Source: CAD feature listing. Evaluate the final solid. Frame: model axes, mm. Face numbers are marked on the shaded views. A direction names the side the tool comes from. Give positions to 0.01 mm unless a question says otherwise; leave off trailing zeros. Loops run counter-clockwise (first coordinate to the right, second up) from the corner with the lowest first, then second, coordinate; pieces in that order, holes last. Notation, with made-up numbers: M 29,-21.75 L 82,-21.75 A32 ccw 82,5.25 Z; hole C -34,45 d1. An arc over 180 degrees is marked long. Write item = value, one per line.
from build123d import *

# Parameters (mm, degrees)
ESQUISSE1_W                              = 45
ESQUISSE1_H                              = 35
BOSS_EXTRU_1_DEPTH                       = 2
ESQUISSE2_W                              = 35
ESQUISSE2_H                              = 32
BOSS_EXTRU_2_DEPTH                       = 1
CONG_1_R                                 = 5
CONG_2_R                                 = 0.5
CHANFREIN1_SIZE                          = 0.5
ESQUISSE3_R                              = 1.75
ENL_V_MAT_EXTRU_1_DEPTH                  = 29.574464124
DIAM_TRE_DU_PER_AGE_6_5_6_5_1_D          = 6.5
DIAM_TRE_DU_PER_AGE_6_5_6_5_1_DEPTH      = 1
FRAISAGE_POUR_VIS_T_TE_FRAIS_E_6_2_COUNT = 2
FRAISAGE_POUR_VIS_T_TE_FRAIS_E_6_2_PITCH = 33.301651611
FRAISAGE_POUR_VIS_T_TE_FRAIS_E_6_3_COUNT = 2
FRAISAGE_POUR_VIS_T_TE_FRAIS_E_6_3_PITCH = 22
FRAISAGE_POUR_VIS_T_TE_FRAIS_E_6_4_COUNT = 2
FRAISAGE_POUR_VIS_T_TE_FRAIS_E_6_4_PITCH = 25


with BuildPart() as part:
    # Esquisse1 → Boss.-Extru.1 (new body)
    with BuildSketch(Plane(origin=(0, 0, 0), x_dir=(1, 0, 0), z_dir=(0, 1, 0))):
        Rectangle(ESQUISSE1_W, ESQUISSE1_H)
    extrude(amount=BOSS_EXTRU_1_DEPTH)

    # Esquisse2 → Boss.-Extru.2 (add)
    with BuildSketch(Plane.XZ):
        Rectangle(ESQUISSE2_W, ESQUISSE2_H)
    extrude(amount=BOSS_EXTRU_2_DEPTH)

    # Congé1
    cong_1_edges = [part.edges().sort_by_distance(p)[0] for p in [
        (17.5, -0.5, -16),
        (17.5, -0.5, 16),
        (-17.5, -0.5, 16),
        (-17.5, -0.5, -16),
    ]]
    fillet(cong_1_edges, radius=CONG_1_R)

    # Congé2
    cong_2_edges = [part.edges().sort_by_distance(p)[0] for p in [
        (22.5, 1, 17.5),
        (-22.5, 1, 17.5),
        (-22.5, 1, -17.5),
        (22.5, 1, -17.5),
    ]]
    fillet(cong_2_edges, radius=CONG_2_R)

    # Chanfrein1
    chanfrein1_edges = [part.edges().sort_by_distance(p)[0] for p in [
        (0, -1, 16),
        (17.5, -1, 0),
        (-17.5, -1, 0),
        (0, -1, -16),
        (-16.035533906, -1, 14.535533906),
        (16.035533906, -1, -14.535533906),
        (-16.035533906, -1, -14.535533906),
        (16.035533906, -1, 14.535533906),
    ]]
    chamfer(chanfrein1_edges, length=CHANFREIN1_SIZE)

    # Esquisse3 → Enlèv. mat.-Extru.1 (cut, through all)
    with BuildSketch(Plane.XZ):
        with Locations(Location((-20, 10, 0), (0, 0, 270))):
            Circle(ESQUISSE3_R)
        with Locations(Location((20, 10, 0), (0, 0, 270))):
            Circle(ESQUISSE3_R)
        with Locations(Location((20, -10, 0), (0, 0, 270))):
            Circle(ESQUISSE3_R)
        with Locations(Location((-20, -10, 0), (0, 0, 270))):
            Circle(ESQUISSE3_R)
    extrude(amount=-ENL_V_MAT_EXTRU_1_DEPTH, mode=Mode.SUBTRACT)

    # Diamètre du perçage Ø6.5 (6.5)1
    with Locations(Plane(origin=(0, 2, 0), x_dir=(1, 0, 0), z_dir=(0, 1, 0))):
        with Locations((-12.5, -11), (12.5, 11), (-12.5, 11), (12.5, -11)):
            Hole(DIAM_TRE_DU_PER_AGE_6_5_6_5_1_D / 2, depth=DIAM_TRE_DU_PER_AGE_6_5_6_5_1_DEPTH)

    # Esquisse4 → Fraisage pour vis à tête fraisée à 6 pans creux M31 (revolve, cut)
    with BuildSketch(Plane(origin=(-12.5, 1, -11), x_dir=(0, 0, 1), z_dir=(1, 0, 0))):
        Polygon((0, 0), (0, 2), (1.7, 2), (1.7, 1.55), (3.25, 0), align=None)
    fraisage_pour_vis_t_te_frais_e_6_pan = revolve(axis=Axis((-12.5, 7.35, -11), (0, -1, 0)), mode=Mode.SUBTRACT)

    # Fraisage pour vis _ t_te frais_e _ 6 2: Fraisage pour vis à tête fraisée à 6 pans creux M31 ×2
    with Locations(*[Vector(0.7507135169227553, 0, 0.6606278948920248) * (i * FRAISAGE_POUR_VIS_T_TE_FRAIS_E_6_2_PITCH) for i in range(1, FRAISAGE_POUR_VIS_T_TE_FRAIS_E_6_2_COUNT)]):
        add(fraisage_pour_vis_t_te_frais_e_6_pan, mode=Mode.SUBTRACT)

    # Fraisage pour vis _ t_te frais_e _ 6 3: Fraisage pour vis à tête fraisée à 6 pans creux M31 ×2
    with Locations(*[(0, 0, i * FRAISAGE_POUR_VIS_T_TE_FRAIS_E_6_3_PITCH) for i in range(1, FRAISAGE_POUR_VIS_T_TE_FRAIS_E_6_3_COUNT)]):
        add(fraisage_pour_vis_t_te_frais_e_6_pan, mode=Mode.SUBTRACT)

    # Fraisage pour vis _ t_te frais_e _ 6 4: Fraisage pour vis à tête fraisée à 6 pans creux M31 ×2
    with Locations(*[(i * FRAISAGE_POUR_VIS_T_TE_FRAIS_E_6_4_PITCH, 0, 0) for i in range(1, FRAISAGE_POUR_VIS_T_TE_FRAIS_E_6_4_COUNT)]):
        add(fraisage_pour_vis_t_te_frais_e_6_pan, mode=Mode.SUBTRACT)


solid = part.part
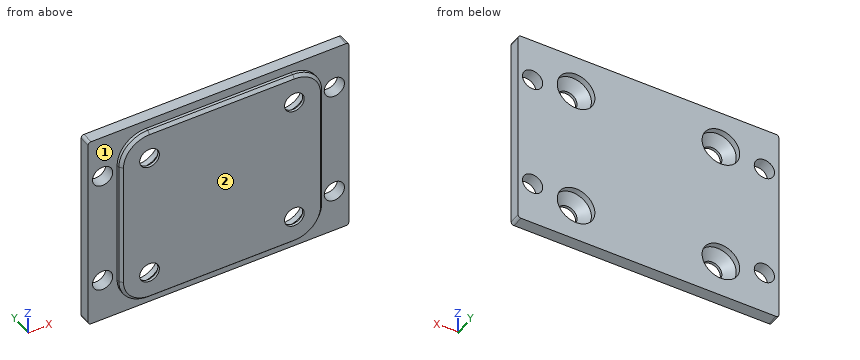
1. Material intervals for probe 1 along Z at (x, y) = (-12.5, -0.75); probe 2 along Z at (x, y) = (-13.5, -0.25); probe 3 along X at (y, z) = (1.6, 10), sorted ascending. Write a range as from..to.
Derived:
probe_1 = -15.75..-12.7, -9.3..9.3, 12.7..15.75
probe_2 = -15.9..-12.73, -9.27..9.27, 12.73..15.9
probe_3 = -22.5..-21.75, -18.25..-15.59, -9.41..9.41, 15.59..18.25, 21.75..22.5
2. Cut plane A-A, the plane x = -20. Return the cut outline in (y, z).
Derived:
outline = M 0,-17.5 L 2,-17.5 L 2,-11.75 L 0,-11.75 Z; M 0,-8.25 L 2,-8.25 L 2,8.25 L 0,8.25 Z; M 0,11.75 L 2,11.75 L 2,17.5 L 0,17.5 Z
3. Cut plane B-B, the plane x = 7. Return the cut outline in (y, z), then the cut area to 3 significant figures.
Derived:
outline = M -1,-15.5 L -0.5,-16 L 0,-16 L 0,-17.5 L 2,-17.5 L 2,17.5 L 0,17.5 L 0,16 L -0.5,16 L -1,15.5 Z
area = 102 mm²
4. First-contact query: pin 1 Ø4 at (x, z) = (20, 10) entering from -Y; pin 2 Ø2 at (x, z) = (-20, -10) entering from +Y; pin 3 Ø10.5 at (x, z) = (12.5, -11) entering from +Y; pin 4 Ø5.5 at (x, z) = (20, -10) entering from -Y. Flat tips, straight axial feed; report the tip coordinate or a pass-through.
Derived:
pin_1 = 0
pin_2 = through
pin_3 = 2
pin_4 = -0.75
5. Cut plane C-C, the plane z = 3. Return the cut outline in (x, y), then the cut area to 3 significant figures.
Derived:
outline = M -22.5,0 L -17.5,0 L -17.5,-0.5 L -17,-1 L 17,-1 L 17.5,-0.5 L 17.5,0 L 22.5,0 L 22.5,2 L -22.5,2 Z
area = 125 mm²
6. Cut plane D-D, the plane z = 10.5. Count the separate pieces of the cut face and the enclosed holes in it, then the cut area to 3 significant figures.
Derived:
separate_pieces = 5
enclosed_holes = 0
area = 80.5 mm²
7. Reachability of the marked faces 1 and 2 from +Z, -Z, +X, -X, +Y, -Y: full face, straight path, thin tool, end or side. Return the list, or none.
Derived:
face_1 = -Y
face_2 = +Z, -Z, +X, -X, -Y
